Solid Edge part; units mm, degrees
sketch "Sketch1" plane through (0, 0, 0) normal (1, 0, 0) x (0, 1, 0)
  line L0 (-108.1482, 2.6153) -> (-28.1482, 2.6153)
  line L1 (-28.1482, 2.6153) -> (-28.1482, 82.6153)
  line L2 (-28.1482, 82.6153) -> (-108.1482, 82.6153)
  line L3 (-108.1482, 82.6153) -> (-108.1482, 2.6153)
  line L4 (-118.1482, -7.3837) -> (-18.1482, -7.3837)
  line L5 (-18.1482, -7.3837) -> (-18.1482, 92.6144)
  line L6 (-18.1482, 92.6144) -> (-118.1482, 92.6163)
  line L7 (-118.1482, 92.6163) -> (-118.1482, -7.3837)
  dimension "D1" = 28.1482
  dimension "D2" = 108.1482
extrude "Protrusion1" add sketch "Sketch1" against normal blind 1850
sketch "Sketch2" plane through (-925, -118.1482, 42.6163) normal (0, -1, 0) x (-1, 0, 0)
  circle A0 centre (-905, -20) radius 4
  circle A1 centre (-865, 20) radius 4
  circle A2 centre (-865, -20) radius 4
  circle A3 centre (-905, 20) radius 4
extrude "Cutout1" cut sketch "Sketch2" against normal through all
mirror "Mirror1" about plane through (-925, -153.5035, -42.739) normal (0, 0.7071, -0.7071) of "Cutout1"
sketch "Sketch3" plane through (-925, -68.1482, -7.3837) normal (0, 0, -1) x (1, 0, 0)
  circle A0 centre (-855, -30) radius 4
  circle A1 centre (-815, 30) radius 4
  circle A2 centre (-815, -30) radius 4
  circle A3 centre (-855, 30) radius 4
extrude "Cutout3" cut sketch "Sketch3" against normal blind 46.6265
properties material "Aluminum, 6061-T6"
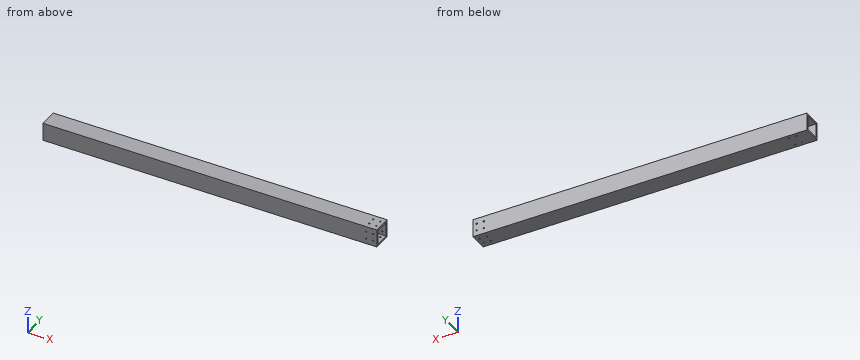
Build history of the part. All positions in model axes, mm. Round coordinates to 2 decimals unless told otherwise and drop trailing zeros. Write each loop counter-clockwise with the first axis right and the second up, starting at its lowest first coordinate (ties: lowest second). Pieces come first, ordered by that corner, then holes. Notation, with made-up numbers: (-4, -39.75) - (1, -39.75) arc R12 ccw to (1, -34.75) - close; hole circle Ø6 at (43.5, -29). An arc over 180 degrees is marked (long way). Use CSV: the item, a comma, the result in double quotes.
(1) Wall check: line 1 (Y direction, x = -20, z = -4); line 2 (Z direction, x = -60, y = -23); line 3 (Y direction, x = -352.5, z = 66). Give the ranges that are in metal, low to high.
Response:
line 1,"-118.15 to -92.15, -84.15 to -52.15, -44.15 to -18.15"
line 2,"-7.38 to 18.62, 26.62 to 58.62, 66.62 to 92.61"
line 3,"-118.15 to -108.15, -28.15 to -18.15"
(2) Band-saw the part on A-A (x = -686). Write the cut outline in (y, z), plus the area to 3 significant figures.
Response:
outline,"(-118.15, -7.38) - (-18.15, -7.38) - (-18.15, 92.61) - (-118.15, 92.62) - close; hole (-108.15, 2.62) - (-28.15, 2.62) - (-28.15, 82.62) - (-108.15, 82.62) - close"
area,"3,600 mm²"
(3) Pin check, flat tips, straight feed: P1, Ø10.5, axis at x = -60, z = 22.62, coming from the -Y side; P2, Ø5, axis at x = -1740, y = -98.15, coming from the -Z side; P3, Ø7, axis at x = -20, z = 62.62, coming from the -Y side (3 decimals). Stop position of each tip, or through.
Response:
P1,"y = -118.15"
P2,"z = 82.62"
P3,"through"
